Autodesk Inventor part; units mm, degrees
ref_plane "YZ Plane" through (0, 0, 0) normal (1, 0, 0) x (0, 1, 0)
ref_plane "XZ Plane" through (0, 0, 0) normal (0, 1, 0) x (-1, 0, 0)
ref_plane "XY Plane" through (0, 0, 0) normal (0, 0, 1) x (1, 0, 0)
ref_plane "Work Plane1" through (0, 0, 0) normal (0, 0, 1) x (1, 0, 0)
sketch "Sketch1" plane through (0, 0, 0) normal (0, 0, 1) x (1, 0, 0)
  arc A0 (-4.3529, 18.17) -> (-4.3529, 17.33) centre (-7.5, 17.75) ccw
  circle A1 centre (-7.5, 17.75) radius 3.175
  point P0 (0, 0)
  dimension "d0" = 6.35
extrude "Extrusion1" add sketch "Sketch1" against normal blind 7.58
sketch "Sketch2" plane through (-7.5, 17.75, 0) normal (0, 0, 1) x (1, 0, 0)
  line L0 (-6.35, -3.425) -> (6.35, -3.425)
  line L1 (6.35, -3.425) -> (6.35, 3.425)
  line L2 (6.35, 3.425) -> (-6.35, 3.425)
  line L3 (-6.35, 3.425) -> (-6.35, -3.425)
  line L4 (-6.35, -3.425) -> (6.35, 3.425) construction
  line L5 (6.35, -3.425) -> (-6.35, 3.425) construction
  point P0 (7.5, -17.75)
  point P1 (0, 0)
  dimension "d3" = 12.7
  dimension "d4" = 6.85
extrude "Extrusion2" add sketch "Sketch2" along normal blind 10.5
sketch "Sketch3" plane through (-7.5, 17.75, -7.58) normal (0, 0, -1) x (-1, 0, 0)
  circle A0 centre (0, 0) radius 2.6
  point P0 (-7.5, -17.75)
  dimension "d7" = 5.2
extrude "Extrusion3" cut sketch "Sketch3" against normal blind 4
sketch "Sketch4" plane through (-7.5, 17.75, -3.58) normal (0, 0, -1) x (-1, 0, 0)
  circle A0 centre (0, 0) radius 1.1094
  point P0 (-7.5, -17.75)
extrude "Extrusion4" add sketch "Sketch4" along normal blind 12
fillet "Fillet1" radius 1 1 edges at (-6.3906, 17.75, -15.58)
thread "Thread1"
chamfer "Chamfer1" distance 1 angle 45 1 edges at (-4.9, 17.75, -3.58)
properties part number "AST13SEBQ"
Read the model definition and answer for the solid it produces. Units are mm, in the model's axes. A direction names the side the tool comes from. Coordinates: 2 decimals unless noted, no trailing zeros. Loops run counter-clockwise (first coordinate to the right, second up) from the corner with the lowest first, then second, coordinate; pieces in that order, holes last.
(1) The part is cut by section C-C (z = -9.25). Determine the outline of the cut face in (x, y), and give its area (3 significant figures).
Solution:
outline: circle Ø2.22 at (-7.5, 17.75)
area: 3.87 mm2
(2) Consider line 1 along Y through (x, z) = (-7.5, -5.15) (3 decimals); line 2 along Y through (x, z) = (-6.5, -7); line 3 along Z through (x, y) = (-9.75, 19.5). Determine where each line is inside the solid, lowest interval first.
Solution:
line 1: y = 14.575 to 15.15, 16.641 to 18.859, 20.35 to 20.925
line 2: y = 14.74 to 15.35, 17.27 to 18.23, 20.15 to 20.76
line 3: z = -7.58 to 10.5
(3) The part is cut by section B-B (x = -12.5). Determine the outline of the cut face in (y, z) (3 decimals).
Solution:
outline: (14.325, 0) - (21.175, 0) - (21.175, 10.5) - (14.325, 10.5) - close
(4) A tool of negligible diameter and unlimited length cuts with its end or side. For faces 4 (the face through (-7, 21.175, 5)), 5 (the face through (-9.98, 18.53, -6.1)), from which of +Z, -Z, +X, -X, +Y, -Y can it reach the whole face along a straight path? Write none if from no direction.
Solution:
face 4: +Z, -Z, +X, -X, +Y
face 5: -Z
(5) The part is cut by section A-A (z = -6.25). Determine the outline of the cut face in (x, y) (3 decimals), and give its area (3 significant figures).
Solution:
outline: circle Ø2.219 at (-7.5, 17.75); (-4.353, 17.33) arc R3.175 ccw to (-4.353, 18.17) arc R3.175 ccw (long way) to start; hole circle Ø5.2 at (-7.5, 17.75)
area: 14.3 mm2
(6) Flat-ended cylindrical pins translate along their axes: pin 1 Ø2 at (x, y) = (-3.5, 16) entering from -Z; pin 2 Ø3.5 at (x, y) = (-9, 19.5) entering from -Z; pin 3 Ø3.5 at (x, y) = (-7.5, 18) entering from -Z. Find the tip coordinate at first contact, or state that the pin passes through.
Solution:
pin 1: stops at z = 0
pin 2: stops at z = -15.48
pin 3: stops at z = -15.58
(7) The mould has two halves that part along Y. Classify faces 1 (the face through (-8, 14.325, 5)), 2 (the face through (-9, 14.75, 0)), 3 (the face through (-8, 19, -3.58)): released by +Y, released by -Y, zero draft, split by the parting line, or undercut.
Solution:
face 1: released by -Y
face 2: zero draft
face 3: undercut
